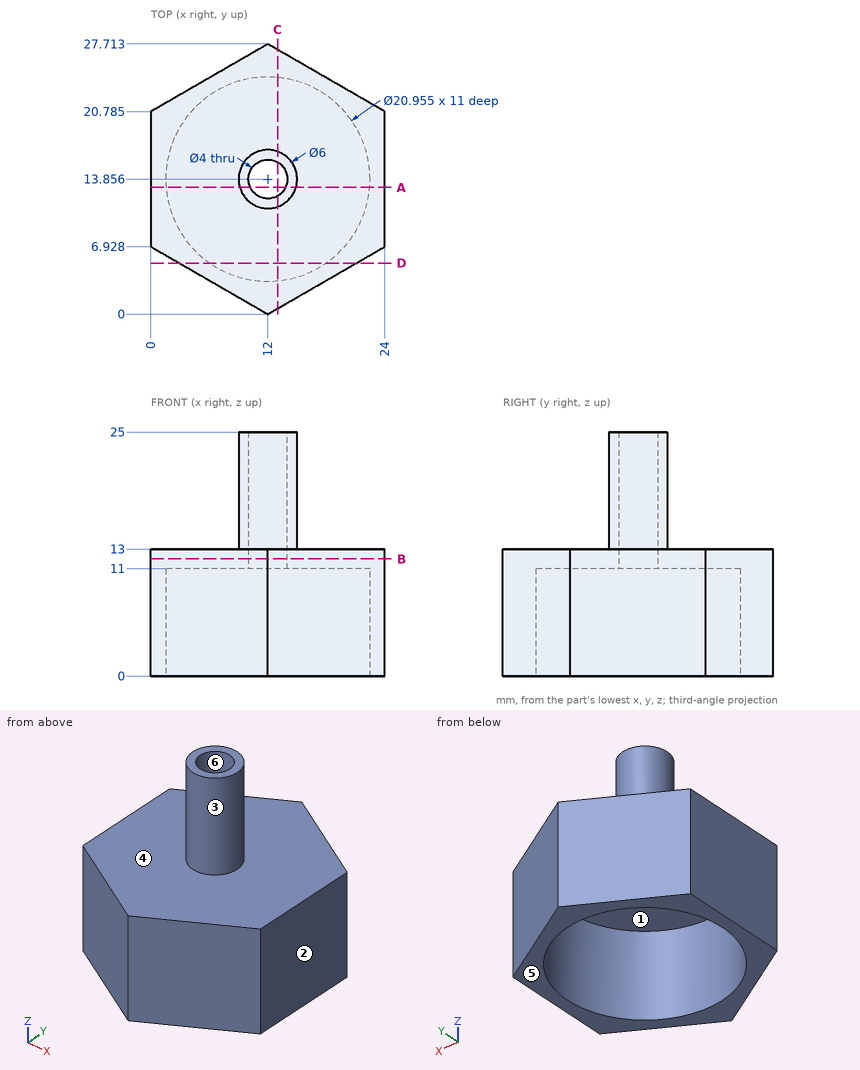
Here's the drawing with two shaded views (mm, measured from the low corner). I have some questions. A direction names the side the tool comes from. Coordinates: 2 decimals unless noted, no trailing zeros. Order: outer loops, then holes, each group sorted by start corner. A loop starts at its lowest first (then second) coordinate and runs counter-clockwise, first axis right, second up.
Item 1: I need wall thicknesses on line 1 (Y direction, x = 12, z = 6.5) (1 decimal); line 2 (Y direction, x = 12, z = 19.5); line 3 (Z direction, x = 3.5, y = 11.75). Which ranges of each line are inside material? Lowest first, please.
Result sheet:
line 1: y = 0 to 3.4, 24.3 to 27.7
line 2: y = 10.86 to 11.86, 15.86 to 16.86
line 3: z = 11 to 13
Item 2: If we mould it in two halves opening along Z, with no side actions, what happens to the marked faces 4, 5 and 6? For each: +Z half, -Z half, draft (parallel to the pull), parting line (faces both ways), or undercut.
Result sheet:
face 4: +Z half
face 5: -Z half
face 6: draft
Item 3: For the marked faces 1, 2 and 3, which set-ups out of +Z, -Z, +X, -X, +Y, -Y let a thin tool reach every point of the face, with its end or its side?
Result sheet:
face 1: -Z
face 2: +Z, -Z, +X, +Y, -Y
face 3: +Z
Item 4: If we section it at C-C on x = 13: List the corners of the cut face in (y, z) for me (1 decimal).
Result sheet:
outline: (0.6, 0) - (3.4, 0) - (3.4, 11) - (12.1, 11) - (12.1, 25) - (11, 25) - (11, 13) - (0.6, 13) - close; (15.6, 11) - (24.3, 11) - (24.3, 0) - (27.1, 0) - (27.1, 13) - (16.7, 13) - (16.7, 25) - (15.6, 25) - close
Item 5: If we section it at D-D on y = 5.25: List the corners of the cut face in (x, z) for me (1 decimal), plus the area to 3 significant figures.
Result sheet:
outline: (2.9, 0) - (6, 0) - (6, 11) - (18, 11) - (18, 0) - (21.1, 0) - (21.1, 13) - (2.9, 13) - close
area: 105 mm2
Item 6: If we section it at A-A on y = 13: List the corners of the cut face in (x, z) for me (1 decimal), plus the area to 3 significant figures.
Result sheet:
outline: (0, 0) - (1.6, 0) - (1.6, 11) - (10.2, 11) - (10.2, 25) - (9.1, 25) - (9.1, 13) - (0, 13) - close; (13.8, 11) - (22.4, 11) - (22.4, 0) - (24, 0) - (24, 13) - (14.9, 13) - (14.9, 25) - (13.8, 25) - close
area: 101 mm2
Item 7: For P1, Ø6.5, axis at x = 9.5, y = 11, coming from the -Z side; P2, Ø4, axis at x = 5, y = 7, coming from the +Z side; P3, Ø1.5, axis at y = 25, z = 14.5, coming from the +X side, each with a flat end and sliding along its axis, tell me the tip position at first contact or that it passes through.
Result sheet:
P1: stops at z = 11
P2: stops at z = 13
P3: passes through
Item 8: If we section it at B-B on z = 12: List the corners of the cut face in (x, y) for me (1 decimal).
Result sheet:
outline: (0, 6.9) - (12, 0) - (24, 6.9) - (24, 20.8) - (12, 27.7) - (0, 20.8) - close; hole circle Ø4 at (12, 13.9)
